Check sheet for the modelled part. Datum: model origin and axes. Units: mm. A direction names the side the tool comes from. Give positions to 0.01 mm unless a question says otherwise; leave off trailing zeros. Order: outer loops, then holes, each group sorted by start corner. A loop starts at its lowest first (then second) coordinate and runs counter-clockwise, first axis right, second up. Notation, with made-up numbers: (-20.5, 71) - (-3.5, 71) arc R24 ccw to (-3.5, 106) - close; hole circle Ø1 at (29, -36.75). An arc over 180 degrees is marked (long way). Answer in a Markdown table with one row per item.
from build123d import *

# Parameters (mm, degrees)
SKETCH_1_R          = 1.25
SKETCH_1_R_2        = 1.8
EXTRUDE_1_DEPTH     = 2
SKETCH_3_R          = 1.8
EXTRUDE_2_DEPTH     = 1.5
SKETCH_4_R          = 2
CUT_EXTRUDE_1_DEPTH = 1
SKETCH_5_W          = 1.6
SKETCH_5_H          = 6
CUT_EXTRUDE_6_DEPTH = 40


with BuildPart() as part:
    # ｽｹｯﾁ1 → ﾎﾞｽ - 押し出し1 (new body)
    with BuildSketch(Plane.XY):
        with BuildLine():
            Line((19.5, -5), (-19.5, -5))
            Line((-19.5, -5), (-19.5, 23))
            Line((-19.5, 23), (-13.5, 23))
            Line((-13.5, 23), (-8.245593322, 15.342245077))
            ThreePointArc((-8.245593322, 15.342245077), (0, 11), (8.245593322, 15.342245077))
            Line((8.245593322, 15.342245077), (13.5, 23))
            Line((13.5, 23), (19.5, 23))
            Line((19.5, 23), (19.5, -5))
        make_face()
        with Locations((-10.5, 0)):
            Circle(SKETCH_1_R, mode=Mode.SUBTRACT)
        with Locations((10.5, 0)):
            Circle(SKETCH_1_R, mode=Mode.SUBTRACT)
        with Locations((-16.25, -1)):
            Circle(SKETCH_1_R_2, mode=Mode.SUBTRACT)
        with Locations((-16.25, 19)):
            Circle(SKETCH_1_R_2, mode=Mode.SUBTRACT)
        with Locations((16.25, -1)):
            Circle(SKETCH_1_R_2, mode=Mode.SUBTRACT)
        with Locations((16.25, 19)):
            Circle(SKETCH_1_R_2, mode=Mode.SUBTRACT)
    extrude(amount=EXTRUDE_1_DEPTH)

    # ｽｹｯﾁ3 → ﾎﾞｽ - 押し出し2 (add)
    with BuildSketch(Plane.XY.offset(2)):
        Polygon((-13, 22.271301653), (-13, -2.6), (13, -2.6), (13, 22.271301653), (13.5, 23), (19.5, 23), (19.5, -5), (-19.5, -5), (-19.5, 23), (-13.5, 23), align=None)
        with Locations((-16.25, 19)):
            Circle(SKETCH_3_R, mode=Mode.SUBTRACT)
        with Locations((-16.25, -1)):
            Circle(SKETCH_3_R, mode=Mode.SUBTRACT)
        with Locations((16.25, -1)):
            Circle(SKETCH_3_R, mode=Mode.SUBTRACT)
        with Locations((16.25, 19)):
            Circle(SKETCH_3_R, mode=Mode.SUBTRACT)
    extrude(amount=EXTRUDE_2_DEPTH)

    # ｽｹｯﾁ4 → ｶｯﾄ - 押し出し1 (cut)
    with BuildSketch(Plane(origin=(0, 0, 0), x_dir=(-1, 0, 0), z_dir=(0, 0, -1))):
        with Locations((-10.5, 0)):
            Circle(SKETCH_4_R)
        with Locations((10.5, 0)):
            Circle(SKETCH_4_R)
    extrude(amount=-CUT_EXTRUDE_1_DEPTH, mode=Mode.SUBTRACT)

    # ｽｹｯﾁ5 → ｶｯﾄ - 押し出し6 (cut, through all)
    with BuildSketch(Plane.ZY.offset(19.5)):
        with Locations((0.8, 5.5)):
            Rectangle(SKETCH_5_W, SKETCH_5_H)
    extrude(amount=-CUT_EXTRUDE_6_DEPTH, mode=Mode.SUBTRACT)


solid = part.part
(1) Thickness scan on L1, parallel to Y at x = -16.25, z = 0.8; L2, parallel to X at y = 0, z = 1.55; L3, parallel to X at y = 1, z = 2.8. Record the ranges inside material, lowest first.
Geometry says:
| item | result |
|---|---|
| L1 | -5 to -2.8, 0.8 to 2.5, 8.5 to 17.2, 20.8 to 23 |
| L2 | -19.5 to -17.75, -14.75 to -11.75, -9.25 to 9.25, 11.75 to 14.75, 17.75 to 19.5 |
| L3 | -19.5 to -13, 13 to 19.5 |
(2) Cross-section at B-B, the plane x = 16.25. Record the cut outline in (y, z).
Geometry says:
| item | result |
|---|---|
| outline | (-5, 0) - (-2.8, 0) - (-2.8, 3.5) - (-5, 3.5) - close; (0.8, 0) - (2.5, 0) - (2.5, 1.6) - (8.5, 1.6) - (8.5, 0) - (17.2, 0) - (17.2, 3.5) - (0.8, 3.5) - close; (20.8, 0) - (23, 0) - (23, 3.5) - (20.8, 3.5) - close |
(3) Cross-section at D-D, the plane y = 9.25. Record the cut outline in (x, z), then the cut area to 3 significant figures.
Geometry says:
| item | result |
|---|---|
| outline | (-19.5, 0) - (19.5, 0) - (19.5, 3.5) - (13, 3.5) - (13, 2) - (-13, 2) - (-13, 3.5) - (-19.5, 3.5) - close |
| area | 97.5 mm² |
(4) Cross-section at A-A, the plane y = 13. Record the cut outline in (x, z), then the cut area to 3 significant figures.
Geometry says:
| item | result |
|---|---|
| outline | (-19.5, 0) - (-6, 0) - (-6, 2) - (-13, 2) - (-13, 3.5) - (-19.5, 3.5) - close; (6, 0) - (19.5, 0) - (19.5, 3.5) - (13, 3.5) - (13, 2) - (6, 2) - close |
| area | 73.5 mm² |
(5) Cross-section at C-C, the plane z = 3. Record the cut outline in (x, y).
Geometry says:
| item | result |
|---|---|
| outline | (-19.5, -5) - (19.5, -5) - (19.5, 23) - (13.5, 23) - (13, 22.27) - (13, -2.6) - (-13, -2.6) - (-13, 22.27) - (-13.5, 23) - (-19.5, 23) - close; hole circle Ø3.6 at (-16.25, -1); hole circle Ø3.6 at (-16.25, 19); hole circle Ø3.6 at (16.25, -1); hole circle Ø3.6 at (16.25, 19) |
(6) Access from +Z, -Z, +X, -X, +Y, -Y to the whole of each face (thin tool, end or side, straight path). Record for faces 4 (the flat face through (0, 7, 2)), 5 (the cylindrical face through (9.25, 0.05, 1.49)), 6 (the cylindrical face through (-8.9, -1.2, 0.5)), 7 (the flat face through (0, 5, 1.6)).
Geometry says:
| item | result |
|---|---|
| face 4 | +Z, +Y |
| face 5 | +Z, -Z |
| face 6 | -Z |
| face 7 | -Z, +X, -X |
(7) Gauge pin test, flat ends, axial feed: P1, Ø3, axis at x = 7, y = 6, coming from the -Z side; P2, Ø8, axis at x = 3, y = -1, coming from the +Z side; P3, Ø3, axis at x = 10.5, y = 0, coming from the +Z side; P4, Ø1.5, axis at y = 4.5, z = 0.5, coming from the +X side. Record the tip position at first contact, or that the pin passes through.
Geometry says:
| item | result |
|---|---|
| P1 | z = 1.6 |
| P2 | z = 3.5 |
| P3 | z = 2 |
| P4 | through |
(8) Mould release check, pull along Y, two halves, no side actions. Record for faces 1 (the flat face through (-13, 10, 3)), 2 (the cylindrical face through (16.016, 20.785, 1.726)), 3 (the flat face through (0, -2.6, 3)): pulls with the +Y half, pulls with the -Y half, needs draft (parallel to the pull), parting line crosses it, or undercut.
Geometry says:
| item | result |
|---|---|
| face 1 | needs draft |
| face 2 | undercut |
| face 3 | pulls with the +Y half |
